CAD build for the part. Positions are in the model's coordinates, mm. Coordinates: 2 decimals unless noted, no trailing zeros. Loops run counter-clockwise (first coordinate to the right, second up) from the corner with the lowest first, then second, coordinate; pieces in that order, holes last.
1) Saw through at A-A, the plane z = 753. Write the cut outline in (x, y).
2) Saw through at C-C, the plane y = -9. Write the cut outline in (x, z).
3) Pin check, flat tip, straight feed: pin 1 Ø12 at (x, z) = (289.5, 838.5) entering from -Y. Stop position of the tip, or through.
4) Wall check: line 1 along Z through (x, y) = (490.5, -30); line 2 along X through (y, z) = (-14.5, 701.5); line 3 along Z through (x, y) = (335.5, -19). Give the ranges that are in metal, low to high.
5) Saw through at B-B, the plane x = 378. Write the cut outline in (y, z).
```python
from build123d import *

# Parameters (mm, degrees)
F0_W     = 580
F0_H     = 1020
F0_W_2   = 490
F0_H_2   = 592.5
F0_H_3   = 292.5
F1_DEPTH = 50
F2_W     = 15
F2_H     = 292.5
F3_DEPTH = 20


with BuildPart() as f1:
    # F0 (on Front) → F1 (new body)
    with BuildSketch(Plane.XZ):
        with Locations((290, 510)):
            Rectangle(F0_W, F0_H)
        with Locations((290, 341.25)):
            Rectangle(F0_W_2, F0_H_2, mode=Mode.SUBTRACT)
        with Locations((290, 828.75)):
            Rectangle(F0_W_2, F0_H_3, mode=Mode.SUBTRACT)
    extrude(amount=F1_DEPTH)

    # F2 (on Front) → F3 (join)
    with BuildSketch(Plane.XZ):
        with Locations((290, 828.75)):
            Rectangle(F2_W, F2_H)
        Polygon((297.5, 637.5), (282.5, 637.5), (282.5, 348.75), (45, 348.75), (45, 333.75), (282.5, 333.75), (282.5, 45), (297.5, 45), (297.5, 333.75), (535, 333.75), (535, 348.75), (297.5, 348.75), align=None)
    extrude(amount=F3_DEPTH)


solid = f1.part
```
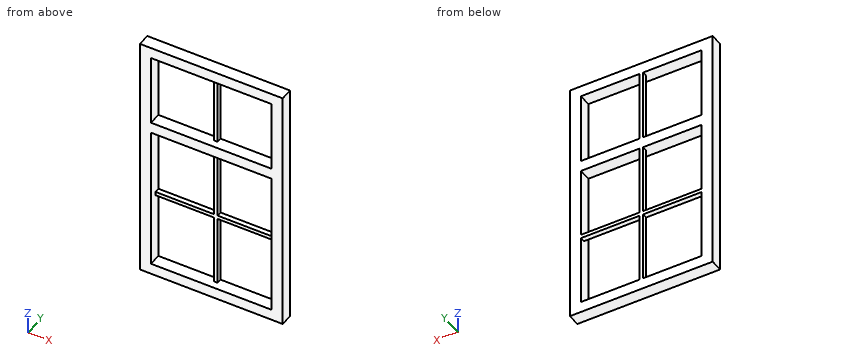
Data:
1. outline: (0, -50) - (45, -50) - (45, 0) - (0, 0) - close; (282.5, -20) - (297.5, -20) - (297.5, 0) - (282.5, 0) - close; (535, -50) - (580, -50) - (580, 0) - (535, 0) - close
2. outline: (0, 0) - (580, 0) - (580, 1020) - (0, 1020) - close; hole (45, 45) - (282.5, 45) - (282.5, 333.75) - (45, 333.75) - close; hole (45, 348.75) - (282.5, 348.75) - (282.5, 637.5) - (45, 637.5) - close; hole (45, 682.5) - (282.5, 682.5) - (282.5, 975) - (45, 975) - close; hole (297.5, 45) - (535, 45) - (535, 333.75) - (297.5, 333.75) - close; hole (297.5, 348.75) - (535, 348.75) - (535, 637.5) - (297.5, 637.5) - close; hole (297.5, 682.5) - (535, 682.5) - (535, 975) - (297.5, 975) - close
3. pin 1: stops at y = -20
4. line 1: z = 0 to 45, 637.5 to 682.5, 975 to 1020
4. line 2: x = 0 to 45, 282.5 to 297.5, 535 to 580
4. line 3: z = 0 to 45, 333.75 to 348.75, 637.5 to 682.5, 975 to 1020
5. outline: (-50, 0) - (0, 0) - (0, 45) - (-50, 45) - close; (-50, 637.5) - (0, 637.5) - (0, 682.5) - (-50, 682.5) - close; (-50, 975) - (0, 975) - (0, 1020) - (-50, 1020) - close; (-20, 333.75) - (0, 333.75) - (0, 348.75) - (-20, 348.75) - close
